Can you work these out from the model? Positions are in its coordinate system, mm. A direction names the side the tool comes from. Give positions to 0.01 mm unless a question says otherwise; leave off trailing zeros. Order: outer loops, then holes, each group sorted by start corner. A loop starts at its lowest first (then second) coordinate and runs counter-clockwise, first axis right, second up. Notation, with made-up numbers: M -19,57 L -1,57 A20 ccw -1,68 Z; hole C 47.5,48.25 d8. An arc over 180 degrees is marked long. Answer as a JSON object with one key per item and string values.
```python
from build123d import *

# Parameters (mm, degrees)
BOSS_EXTRUDE1_DEPTH = 4
SKETCH2_R           = 2.5
CUT_EXTRUDE1_DEPTH  = 22.9089023
SKETCH3_R           = 3
CUT_EXTRUDE2_DEPTH  = 2
CUT_EXTRUDE3_DEPTH  = 1.2
CUT_EXTRUDE5_DEPTH  = 0.7
CUT_EXTRUDE8_START  = -2
CUT_EXTRUDE8_DEPTH  = 2
BOSS_EXTRUDE3_DEPTH = 2
FILLET3_R           = 0.5
CUT_EXTRUDE9_DEPTH  = 2
BOSS_EXTRUDE4_DEPTH = 1.9


with BuildPart() as part:
    # Sketch1 → Boss-Extrude1 (new body)
    with BuildSketch(Plane(origin=(0, 0, 0), x_dir=(1, 0, 0), z_dir=(0, 1, 0))):
        with BuildLine():
            Line((-6.5, -20), (6.5, -20))
            Line((6.5, -20), (6.5, -4.663689527))
            ThreePointArc((6.5, -4.663689527), (8, 0), (6.5, 4.663689527))
            ThreePointArc((6.5, 4.663689527), (0, 8), (-6.5, 4.663689527))
            ThreePointArc((-6.5, 4.663689527), (-8, 0), (-6.5, -4.663689527))
            Line((-6.5, -4.663689527), (-6.5, -20))
        make_face()
    extrude(amount=-BOSS_EXTRUDE1_DEPTH)

    # Sketch2 → Cut-Extrude1 (cut, through all)
    with BuildSketch(Plane(origin=(0, 0, 0), x_dir=(1, 0, 0), z_dir=(0, 1, 0))):
        with Locations(Location((0, 0, 0), (0, 0, 270))):
            Circle(SKETCH2_R)
    extrude(amount=-CUT_EXTRUDE1_DEPTH, mode=Mode.SUBTRACT)

    # Sketch3 → Cut-Extrude2 (cut)
    with BuildSketch(Plane(origin=(0, 0, 0), x_dir=(1, 0, 0), z_dir=(0, 1, 0))):
        with Locations(Location((0, 0, 0), (0, 0, 270))):
            Circle(SKETCH3_R)
    extrude(amount=-CUT_EXTRUDE2_DEPTH, mode=Mode.SUBTRACT)

    # Sketch4 → Cut-Extrude3 (cut)
    with BuildSketch(Plane.XZ.offset(4)):
        Polygon((2.5, -5.75), (-2.5, -5.75), (-5.75, -2.5), (-5.75, 6.25), (-4.4, 6.25), (-4.4, 8.2), (-5.660373569, 10), (-6.5, 10), (-6.5, 11.199110814), (-6.5, 15), (6.5, 15), (6.5, 11.199110814), (6.5, 10), (6.5, 8.2), (4.4, 8.2), (4.4, 6.25), (5.75, 6.25), (5.75, -2.5), align=None)
    extrude(amount=-CUT_EXTRUDE3_DEPTH, mode=Mode.SUBTRACT)

    # Sketch6 → Cut-Extrude5 (cut)
    with BuildSketch(Plane.XZ.offset(2.8)):
        Polygon((6.5, 8.2), (6.5, 15), (-6.5, 15), (-6.5, 11.199110814), (-5.660373569, 10), (-4.4, 8.2), (-4.4, 6.2), (4.4, 6.2), (4.4, 8.2), align=None)
    extrude(amount=-CUT_EXTRUDE5_DEPTH, mode=Mode.SUBTRACT)

    # Sketch10 → Cut-Extrude8 (cut)
    with BuildSketch(Plane.XZ.offset(4).offset(CUT_EXTRUDE8_START)):
        with BuildLine():
            Line((-6.5, 4.663689527), (-6.5, -2.5))
            Line((-6.5, -2.5), (-7.599342077, -2.5))
            ThreePointArc((-7.599342077, -2.5), (-7.907431546, 1.213476964), (-6.5, 4.663689527))
        make_face()
        with BuildLine():
            Line((6.5, 4.663689527), (6.5, -2.5))
            Line((6.5, -2.5), (7.599342077, -2.5))
            ThreePointArc((7.599342077, -2.5), (7.907431546, 1.213476964), (6.5, 4.663689527))
        make_face()
    extrude(amount=CUT_EXTRUDE8_DEPTH, mode=Mode.SUBTRACT)

    # Sketch11 → Boss-Extrude3 (add)
    with BuildSketch(Plane.XZ.offset(4)):
        with BuildLine():
            Line((-0.75, -7.964766161), (-0.75, -5.75))
            Line((-0.75, -5.75), (-2.5, -5.75))
            Line((-2.5, -5.75), (-4.125, -4.125))
            Line((-4.125, -4.125), (-5.656854249, -5.656854249))
            ThreePointArc((-5.656854249, -5.656854249), (-3.404931672, -7.239229262), (-0.75, -7.964766161))
        make_face()
        with BuildLine():
            Line((0.75, -7.964766161), (0.75, -5.75))
            Line((0.75, -5.75), (2.5, -5.75))
            Line((2.5, -5.75), (4.125, -4.125))
            Line((4.125, -4.125), (5.656854249, -5.656854249))
            ThreePointArc((5.656854249, -5.656854249), (3.404931672, -7.239229262), (0.75, -7.964766161))
        make_face()
    extrude(amount=BOSS_EXTRUDE3_DEPTH)

    # Fillet3
    fillet3_edges = [part.edges().sort_by_distance(p)[0] for p in [
        (0, -2, -3),
    ]]
    fillet(fillet3_edges, radius=FILLET3_R - 0.0001)  # a hair under: the kernel refuses the full size

    # Sketch12 → Cut-Extrude9 (cut)
    with BuildSketch(Plane.XZ.offset(4)):
        Polygon((0, 15), (1.5, 15), (1.5, 20), (-1.5, 20), (-1.5, 15), align=None)
    extrude(amount=-CUT_EXTRUDE9_DEPTH, mode=Mode.SUBTRACT)

    # Sketch13 → Boss-Extrude4 (add)
    with BuildSketch(Plane.XZ.offset(2.1)):
        Polygon((-6.5, 15), (-6.5, 10), (-5.660373569, 10), (-4.4, 8.2), (-4.4, 15), align=None)
    extrude(amount=BOSS_EXTRUDE4_DEPTH)


solid = part.part
```
1) I want a section at C-C on z = 5.25. Write out the boundary of the cut face in (x, y).
Results found:
{"outline": "M -6.5,-4 L -5.75,-4 L -5.75,-2.8 L 5.75,-2.8 L 5.75,-4 L 6.5,-4 L 6.5,0 L -6.5,0 Z"}
2) I want a section at B-B on y = -3.6. Write out the boundary of the cut face in (x, z).
Results found:
{"outline": "M -7.6,-2.5 A8 ccw 7.6,-2.5 L 6.5,-2.5 L 6.5,8.2 L 4.4,8.2 L 4.4,6.25 L 5.75,6.25 L 5.75,-2.5 L 2.5,-5.75 L -2.5,-5.75 L -5.75,-2.5 L -5.75,6.25 L -4.4,6.25 L -4.4,15 L -1.5,15 L -1.5,20 L -6.5,20 L -6.5,-2.5 Z; M 1.5,15 L 6.5,15 L 6.5,20 L 1.5,20 Z"}
3) I need wall thicknesses on L1, parallel to X at y = -2.4, z = 0; L2, parallel to X at y = -1, z = 0; L3, parallel to X at y = -1.2, z = 11.75. Which ranges of each line are inside material? Lowest first, please.
Results found:
{"L1": "x = -6.5 to -2.5, 2.5 to 6.5", "L2": "x = -8 to -3, 3 to 8", "L3": "x = -6.5 to 6.5"}
4) I'm going to push flat-ended pins straight in: pin 1 Ø0.6 at (x, y) = (4, -3.5) entering from -Z; pin 2 Ø0.6 at (y, z) = (-3.5, 17.5) entering from -X; pin 3 Ø4.5 at (x, z) = (0, 0) entering from -Y; pin 4 Ø0.5 at (x, y) = (-7, -2.5) entering from +Z. Where does each tip first touch, or does it pass through?
Results found:
{"pin 1": "stops at z = -7.09", "pin 2": "stops at x = -6.5", "pin 3": "passes through", "pin 4": "stops at z = -2.5"}
5) Thinking about a two-plate mould opening in X: for faces 6 (the face through (5, -3, 6.25)), 7 (the face through (-3, -6, -6)), 8 (the face through (-5, -5, -5)), which applies, pulls with the +X half, pulls with the -X half, needs draft (parallel to the pull), parting line crosses it, or undercut?
Results found:
{"face 6": "undercut", "face 7": "needs draft", "face 8": "pulls with the -X half"}
6) I want a section at D-D on y = -0.7. Write out the boundary of the cut face in (x, z), and give its area (3 significant figures).
Results found:
{"outline": "M -6.5,4.66 A8 ccw long 6.5,4.66 L 6.5,20 L -6.5,20 Z; hole C 0,0 d6", "area": "342 mm²"}
7) For faces 1 (the face through (4.4, -3, 7)), 2 (the face through (-7, -3, -2.5)), 3 (the face through (7, -3, -2.5)), 4 (the face through (-3, -3, 15)), 5 (the face through (0, -2, 18)), which set-ups out of +Z, -Z, +X, -X, +Y, -Y let a thin tool reach every point of the face, with its end or its side?
Results found:
{"face 1": "-Y", "face 2": "+Z, -X, -Y", "face 3": "+Z, +X, -Y", "face 4": "+X, -Y", "face 5": "+Z, -Y"}
